Here's how the part is built. I have some questions about the finished solid (model axes, mm). Face numbers are marked on the shaded views. A direction names the side the tool comes from. Give positions to 0.01 mm unless a question says otherwise; leave off trailing zeros. Loops run counter-clockwise (first coordinate to the right, second up) from the corner with the lowest first, then second, coordinate; pieces in that order, holes last. Notation, with made-up numbers: (-10, 76.5) -> (7, 76.5) arc R24 cw to (7, 112.5) -> close; hole circle Ø7 at (52.25, 69.5). An arc over 180 degrees is marked (long way). Answer in a Markdown table with one row per item. Add a question column.
Item 1: If I drill on line 1 (Y direction, x = -10, z = -14.05); line 2 (Y direction, x = -10, z = -14.4); line 3 (X direction, y = -18, z = -14.05), over which ranges is the centre line in solid material (lowest first)?
Item 2: If we section it at D-D (y = -6): Write out the boundary of the cut face in (x, z), then the cut area to 3 significant figures.
Item 3: We'd pull the mould along X, two halves only. Please class the marked faces 3, 4 and 5: released by +X, released by -X, zero draft, split by the parting line, or undercut.
Item 4: If we section it at B-B (y = -18): Write out the boundary of the cut face in (x, z), then the cut area to 3 significant figures.
Item 5: If we section it at C-C (x = -10): Write out the boundary of the cut face in (y, z), then the cut area to 3 significant figures.
Item 6: For P1, Ø1.2, axis at x = -10, y = -5.5, coming from the -Z side, with a flat end and sliding along its axis, tell me the tip position at first contact or that it passes through.
Item 7: If we section it at A-A (z = -13.7): Write out the boundary of the cut face in (x, y), then the cut area to 3 significant figures.
Item 8: Which directions (+Z, -Z, +X, -X, +Y, -Y) give clear straight access to the entire face, cutting with the end or side of a thin tool? Please do the marked faces 1 and 2.
```python
from build123d import *

# Parameters (mm, degrees)
CYLINDER047_R          = 0.75
CYLINDER047_DEPTH      = 10
CYLINDER046_R          = 0.75
CYLINDER046_DEPTH      = 10
BOX034_W               = 4
BOX034_H               = 19
BOX034_DEPTH           = 5
FILLET008_R            = 1
FILLET009_R            = 1
FILLET010_R            = 1
FILLET011_R            = 1
CUT066_PLACEMENT_ANGLE = 180


with BuildPart() as cilindro047:
    # Cylinder047 → Cylinder047 (new body)
    with BuildSketch(Plane(origin=(-39, 66, 48), x_dir=(1, 0, 0), z_dir=(0, 0, 1))):
        Circle(CYLINDER047_R)
    extrude(amount=CYLINDER047_DEPTH)


with BuildPart() as cilindro046:
    # Cylinder046 → Cylinder046 (new body)
    with BuildSketch(Plane(origin=(-39, 53, 48), x_dir=(1, 0, 0), z_dir=(0, 0, 1))):
        Circle(CYLINDER046_R)
    extrude(amount=CYLINDER046_DEPTH)


with BuildPart() as cut066:
    # Box034 → Box034 (new body)
    with BuildSketch(Plane(origin=(-2, 50, 45), x_dir=(1, 0, 0), z_dir=(0, 0, 1))):
        with Locations((2, 9.5)):
            Rectangle(BOX034_W, BOX034_H)
    extrude(amount=BOX034_DEPTH)

    # Fillet008
    fillet008_edges = [cut066.edges().sort_by_distance(p)[0] for p in [
        (2, 59.5, 50),
    ]]
    fillet(fillet008_edges, radius=FILLET008_R)

    # Fillet009
    fillet009_edges = [cut066.edges().sort_by_distance(p)[0] for p in [
        (-2, 59.5, 50),
    ]]
    fillet(fillet009_edges, radius=FILLET009_R)

    # Fillet010
    fillet010_edges = [cut066.edges().sort_by_distance(p)[0] for p in [
        (0, 69, 50),
    ]]
    fillet(fillet010_edges, radius=FILLET010_R)

    # Fillet011
    fillet011_edges = [cut066.edges().sort_by_distance(p)[0] for p in [
        (0, 50, 50),
    ]]
    fillet(fillet011_edges, radius=FILLET011_R)


with BuildPart() as cut066_1:
    # Fillet011 placement: moved
    add(cut066.part.moved(Location((-39, 0, 0))))

    # Cut065: cut Cilindro046
    add(cilindro046.part, mode=Mode.SUBTRACT)

    # Cut066: cut Cilindro047
    add(cilindro047.part, mode=Mode.SUBTRACT)


with BuildPart() as cut066_2:
    # Cut066 placement: moved
    add(cut066_1.part.moved(Location((-49, -71, 35))).rotate(Axis((-49, -71, 35), (0, 1, 0)), CUT066_PLACEMENT_ANGLE))


solid = cut066_2.part
```
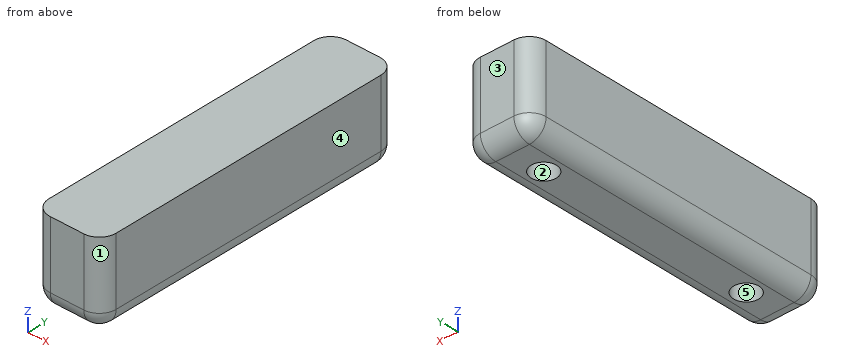
Recorded:
| question | item | result |
|---|---|---|
| 1 | line 1 | y = -21 to -18.75, -17.25 to -5.75, -4.25 to -2 |
| 1 | line 2 | y = -20.92 to -18.75, -17.25 to -5.75, -4.25 to -2.08 |
| 1 | line 3 | x = -12 to -10.75, -9.25 to -8 |
| 2 | outline | (-12, -14) arc R1 ccw to (-11, -15) -> (-9, -15) arc R1 ccw to (-8, -14) -> (-8, -10) -> (-12, -10) -> close |
| 2 | area | 19.6 mm^2 |
| 3 | face 3 | zero draft |
| 3 | face 4 | released by +X |
| 3 | face 5 | undercut |
| 4 | outline | (-12, -14) arc R1 ccw to (-11, -15) -> (-10.75, -15) -> (-10.75, -13) -> (-9.25, -13) -> (-9.25, -15) -> (-9, -15) arc R1 ccw to (-8, -14) -> (-8, -10) -> (-12, -10) -> close |
| 4 | area | 16.6 mm^2 |
| 5 | outline | (-21, -14) arc R1 ccw to (-20, -15) -> (-18.75, -15) -> (-18.75, -13) -> (-17.25, -13) -> (-17.25, -15) -> (-5.75, -15) -> (-5.75, -13) -> (-4.25, -13) -> (-4.25, -15) -> (-3, -15) arc R1 ccw to (-2, -14) -> (-2, -10) -> (-21, -10) -> close |
| 5 | area | 88.6 mm^2 |
| 6 | P1 | stops at z = -15 |
| 7 | outline | (-12, -20) arc R1 ccw to (-11, -21) -> (-9, -21) arc R1 ccw to (-8, -20) -> (-8, -3) arc R1 ccw to (-9, -2) -> (-11, -2) arc R1 ccw to (-12, -3) -> close; hole circle Ø1.5 at (-10, -18); hole circle Ø1.5 at (-10, -5) |
| 7 | area | 71.6 mm^2 |
| 8 | face 1 | +Z, -Z, +X, -Y |
| 8 | face 2 | -Z |
